Input: part model. Units: mm. Frame: model coordinates. Coordinates: 2 decimals unless noted, no trailing zeros. Write each loop counter-clockwise with the first axis right and the second up, starting at its lowest first coordinate (ties: lowest second). Pieces come first, ordered by that corner, then holes. Notation, with made-up numbers: M 13.25,-9 L 36.25,-9 A21 cw 36.25,20 Z; hole C -15,39 d1. An arc over 180 degrees is marked long. Use CSV: the item, a comma, the result in double quotes.
```python
from build123d import *

# Parameters (mm, degrees)
SKETCH1_W                             = 63.5
SKETCH1_H                             = 12.7
F_1_4_0_25_DIAMETER_HOLE1_D           = 6.35
F_1_4_0_25_DIAMETER_HOLE1_CSINK_D     = 7.62
F_1_4_0_25_DIAMETER_HOLE1_CSINK_ANGLE = 90
CIRPATTERN1_COUNT                     = 12


with BuildPart() as part:
    # Sketch1 → Revolve1 (revolve)
    with BuildSketch(Plane.XY):
        with Locations((-95.25, -6.35)):
            Rectangle(SKETCH1_W, SKETCH1_H)
    revolve(axis=Axis((0, 0, 0), (0, 1, 0)))

    # 1/4 (0.25) Diameter Hole1 (through all)
    with Locations(Plane(origin=(114.3, 0, 0), x_dir=(0, 0, 1), z_dir=(0, 1, 0))):
        with Locations((0, 0)):
            f_1_4_0_25_diameter_hole1 = CounterSinkHole(F_1_4_0_25_DIAMETER_HOLE1_D / 2, F_1_4_0_25_DIAMETER_HOLE1_CSINK_D / 2, counter_sink_angle=F_1_4_0_25_DIAMETER_HOLE1_CSINK_ANGLE)

    # CirPattern1: 1/4 (0.25) Diameter Hole1 ×12 about axis
    cirpattern1_axis = Axis((0, 0, 0), (0, 1, 0))
    for i in range(1, CIRPATTERN1_COUNT):
        add(f_1_4_0_25_diameter_hole1.rotate(cirpattern1_axis, i * 360 / CIRPATTERN1_COUNT), mode=Mode.SUBTRACT)


solid = part.part
```
1. Section B-B (x = -42). Return loops of the section in (y, z).
Resolved:
outline,"M -12.7,-119.85 L 0,-119.85 L 0,-47.63 L -12.7,-47.63 Z; M -12.7,47.63 L 0,47.63 L 0,119.85 L -12.7,119.85 Z"
2. Section D-D (z = 21). Return loops of the section in (x, y).
Resolved:
outline,"M -125.25,-12.7 L -59.93,-12.7 L -59.93,0 L -125.25,0 Z; M 59.93,-12.7 L 125.25,-12.7 L 125.25,0 L 59.93,0 Z"
3. Section A-A (z = 114.3). Return loops of the section in (x, y) (3 decimals).
Resolved:
outline,"M -55.358,-12.7 L -3.175,-12.7 L -3.175,-0.635 L -3.81,0 L -55.358,0 Z; M 3.175,-12.7 L 55.358,-12.7 L 55.358,0 L 3.81,0 L 3.175,-0.635 Z"
4. Mould query, pull axis Z, two halves, no side actions, for faces 1 (the cylindrical face through (0.69, -6.75, -111.2)), 2 (the flat face through (-26.4, -12.7, 58.2)). Classes: pulls with the +Z half, pulls with the -Z half, needs draft (parallel to the pull), parting line crosses it, or undercut.
Resolved:
face 1,"undercut"
face 2,"needs draft"
5. Section C-C (y = -10.25). State how many separate pieces and enclosed holes the cut face has, then the cut area to 3 significant figures.
Resolved:
separate pieces,"1"
enclosed holes,"13"
area,"37,600 mm^2"
6. Material intervals for line 1 (X direction, y = -9.25, z = -2.5); line 2 (Z direction, x = 57, y = -1.5); line 3 (X direction, y = -9, z = -2), sorted ascending. Write a range as [from, to].
Resolved:
line 1,"x = [-126.98, -116.26], [-112.34, -63.45], [63.45, 112.34], [116.26, 126.98]"
line 2,"z = [-113.49, -102.16], [-95.82, -27.99], [27.99, 95.82], [102.16, 113.49]"
line 3,"x = [-126.98, -116.77], [-111.83, -63.47], [63.47, 111.83], [116.77, 126.98]"
7. Contact query for flat-ended pins moving along their axis: pin 1 Ø7.5 at (x, z) = (-57.15, 98.99) entering from +Y; pin 2 Ø6 at (x, y) = (-86.5, -5) entering from -Z; pin 3 Ø1.5 at (y, z) = (-3, -83) entering from +X. Output: stop coordinate, or through.
Resolved:
pin 1,"stops at y = -0.06"
pin 2,"stops at z = -95.69"
pin 3,"stops at x = 96.77"
